The figure shows three views and two pictorial views of one solid part (mm, origin at its lowest corner). Answer the questions. Give positions to 0.01 mm unless a question says otherwise; leave off trailing zeros. Write each loop counter-clockwise with the first axis right and the second up, starting at its lowest first coordinate (ties: lowest second). Pieces come first, ordered by that corner, then holes. Notation, with made-up numbers: M -30,-2 L 27,-2 A35 cw 27,32 Z; hole C -26,58 d3. An arc over 180 degrees is marked long. Return JSON: item names as keys, results as strings.
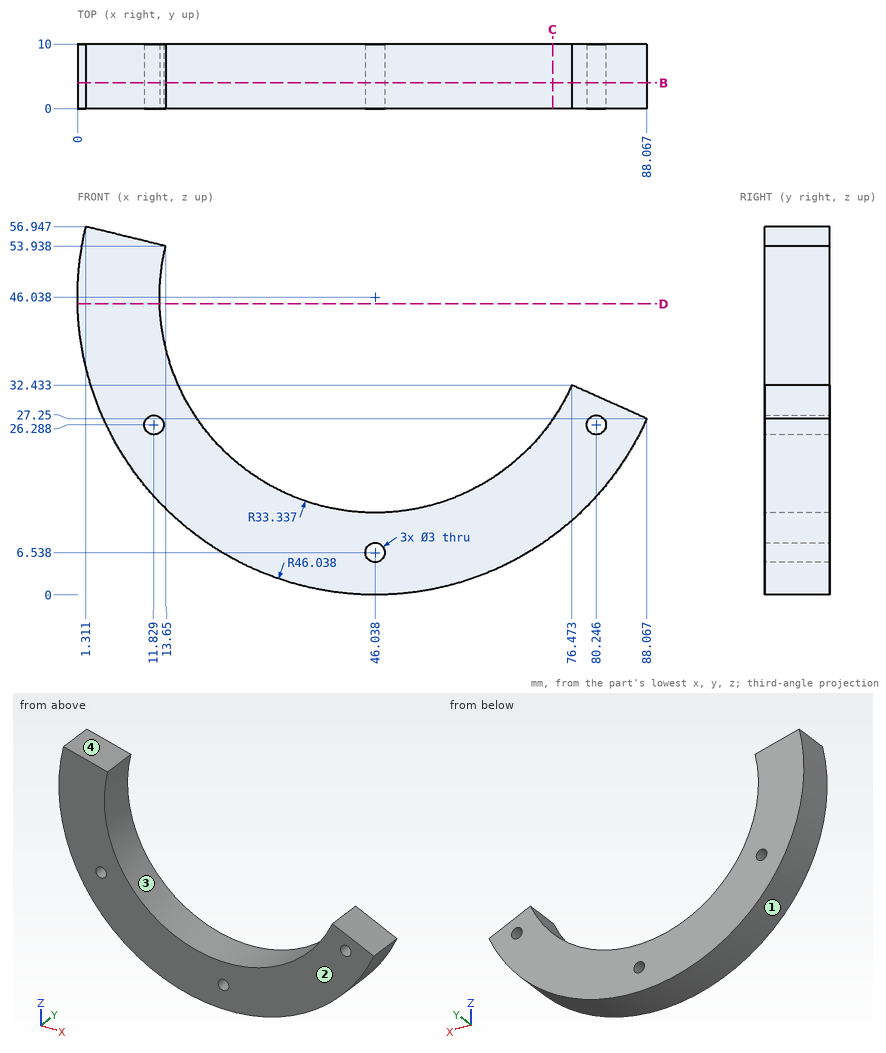
Item 1: A cutting plane is placed at B-B, the plane y = 4. Count the separate pieces of the cut face and the enclosed holes in it, plus the area to 3 significant figures.
Geometry results:
{"separate pieces": "1", "enclosed holes": "3", "area": "1,470 mm2"}
Item 2: A cutting plane is placed at D-D, the plane z = 45. Write down the section's boundary in (x, y).
Geometry results:
{"outline": "M 0.01,0 L 12.72,0 L 12.72,10 L 0.01,10 Z"}
Item 3: Find the intervals of material crossed by line 1 (Z direction, x = 12.5, y = 7) (1 decimal); line 2 (X direction, y = 9, z = 5) (1 decimal); line 3 (X direction, y = 8.75, z = 31.5) (1 decimal), in increasing order.
Geometry results:
{"line 1": "z = 14.5 to 24.9, 27.6 to 54.2", "line 2": "x = 25.2 to 66.9", "line 3": "x = 2.4 to 16, 76 to 78.6"}
Item 4: Given pin 1 Ø3 at (y, z) = (8, 30) entering from +X (1 decimal); pin 2 Ø1.5 at (x, y) = (32, 3.5) entering from -Z; pin 3 Ø1.5 at (x, y) = (26, 6) entering from -Z (1 decimal), each flat-ended and moving along its own axis, determine where each tip first touches the part or whether it passes through.
Geometry results:
{"pin 1": "stops at x = 85.3", "pin 2": "stops at z = 1.96", "pin 3": "stops at z = 4.2"}
Item 5: Determine the mould class of the marked faces 1, 2, 3 and 4 for opening direction X: +X half, -X half, draft (parallel to the pull), parting line (faces both ways), or undercut.
Geometry results:
{"face 1": "parting line", "face 2": "draft", "face 3": "undercut", "face 4": "+X half"}
Item 6: A cutting plane is placed at C-C, the plane x = 73.5. Write down the section's boundary in (y, z).
Geometry results:
{"outline": "M 0,9.09 L 10,9.09 L 10,27.14 L 0,27.14 Z"}
